from build123d import *

# Parameters (mm, degrees)
F0_W     = 150
F0_H     = 140
F1_DEPTH = 4
F2_W     = 4
F2_H     = 10
F3_DEPTH = 4


with BuildPart() as f1:
    # F0 (on Top) → F1 (new body)
    with BuildSketch(Plane.XY):
        Rectangle(F0_W, F0_H)
    extrude(amount=F1_DEPTH)

    # F2 (on face) → F3 (join)
    with BuildSketch(Plane.XY.offset(4)):
        with Locations((-77, -60)):
            Rectangle(F2_W, F2_H)
        with Locations((-77, -40)):
            Rectangle(F2_W, F2_H)
        with Locations((-77, -20)):
            Rectangle(F2_W, F2_H)
        with Locations((-77, 0)):
            Rectangle(F2_W, F2_H)
        with Locations((-77, 20)):
            Rectangle(F2_W, F2_H)
        with Locations((-77, 40)):
            Rectangle(F2_W, F2_H)
        with Locations((-77, 60)):
            Rectangle(F2_W, F2_H)
        with Locations((77, 0)):
            Rectangle(F2_W, F2_H)
        with Locations((77, 60)):
            Rectangle(F2_W, F2_H)
        with Locations((77, 20)):
            Rectangle(F2_W, F2_H)
        with Locations((77, -40)):
            Rectangle(F2_W, F2_H)
        with Locations((77, -60)):
            Rectangle(F2_W, F2_H)
        with Locations((77, -20)):
            Rectangle(F2_W, F2_H)
        with Locations((77, 40)):
            Rectangle(F2_W, F2_H)
    extrude(amount=-F3_DEPTH)


solid = f1.part
CAD build for the part. Positions are in the model's coordinates, mm. A direction names the side the tool comes from. Give positions to 0.01 mm unless a question says otherwise; leave off trailing zeros. Write each loop counter-clockwise with the first axis right and the second up, starting at its lowest first coordinate (ties: lowest second). Pieces come first, ordered by that corner, then holes. Notation, with made-up numbers: M 30,49.25 L 83,49.25 A11 ccw 83,64.25 Z; hole C 25.5,26.5 d9. An arc over 180 degrees is marked long. Put each result on its own line as item: value. Start each with the question number.
(1) Flat gauge pins, fed straight in: pin 1 Ø1.2 at (x, z) = (76, 2.5) entering from +Y; pin 2 Ø1.2 at (x, z) = (77.5, 1.5) entering from -Y; pin 3 Ø2 at (y, z) = (51, 3) entering from +X. Where does each tip first touch, or does it go through?
(2) Mould opens along Y. For faces 4 (the face through (-77, -15, 2)), 5 (the face through (79, 0, 2)), 6 (the face through (77, 65, 2)) say: +Y half, -Y half, draft (parallel to the pull), parting line (faces both ways), or undercut.
(3) Band-saw the part on A-A, the plane y = -52.5. Write the cut outline in (x, z).
(4) Which spindle directions (+Z, -Z, +X, -X, +Y, -Y) get a long thin tool onto all of the face, cutting with end or side? Do faces 1 (the face through (77, -15, 2)), 2 (the face through (-1, 1, 4)), 3 (the face through (-77, 55, 2)). Say none if no direction does.
(5) Probe L1, parallel to X at y = -34, z = 3.55. List the from-to ranges inside material, lowest first.
Response values:
1. pin 1: stops at y = 65
1. pin 2: stops at y = -65
1. pin 3: stops at x = 75
2. face 4: undercut
2. face 5: draft
2. face 6: +Y half
3. outline: M -75,0 L 75,0 L 75,4 L -75,4 Z
4. face 1: +Z, -Z, +X
4. face 2: +Z, +X, -X, +Y, -Y
4. face 3: +Z, -Z, -X
5. L1: x = -75 to 75
